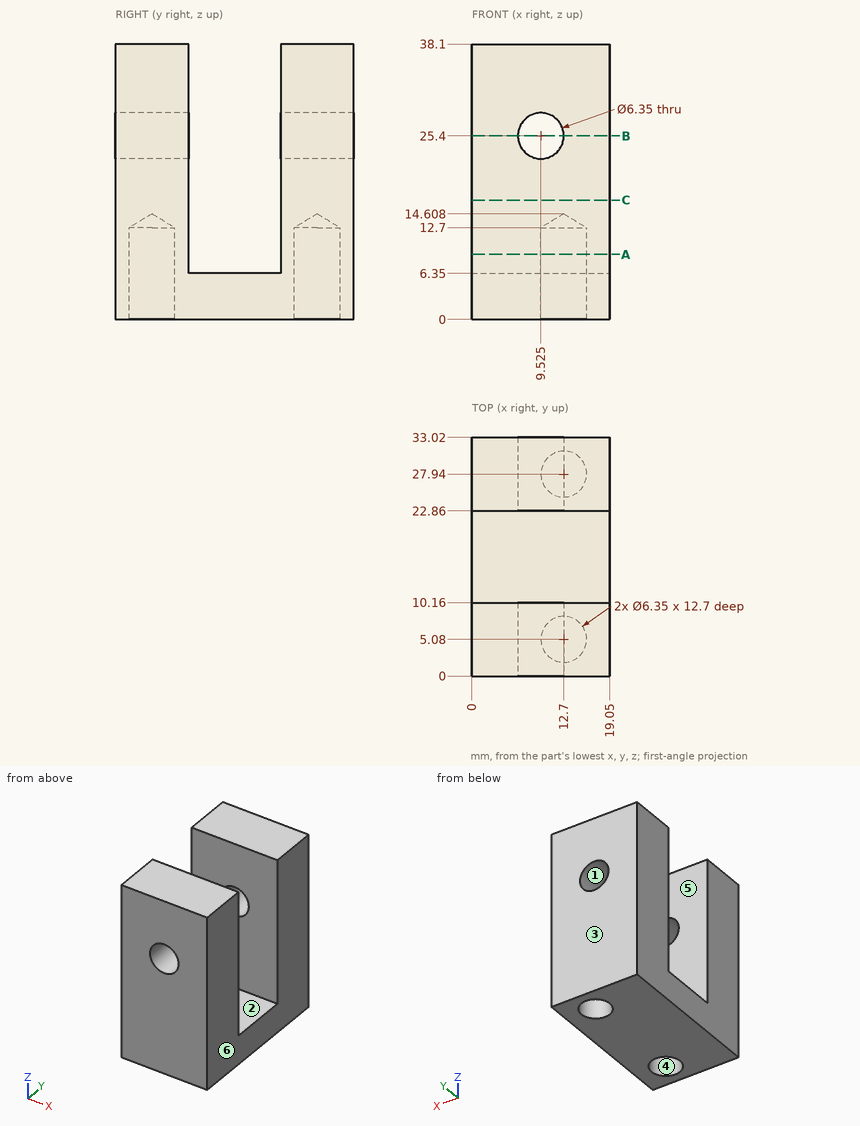
The figure shows three views and two pictorial views of one solid part (mm, origin at its lowest corner). Answer the questions. A direction names the side the tool comes from. Round coordinates to 2 decimals unless told otherwise and drop trailing zeros. Loops run counter-clockwise (first coordinate to the right, second up) from the corner with the lowest first, then second, coordinate; pieces in that order, holes last. Notation, with made-up numbers: (83.25, 63.5) - (136.25, 63.5) arc R19 ccw to (136.25, 71.5) - close; hole circle Ø1 at (42, 33). An arc over 180 degrees is marked (long way). Use one line per item in the form item = value. Start each with the question number.
(1) Find section A-A on z = 9. Give the number of separate pieces and of enclosed holes in the cut face, and give its area (3 significant figures).
(2) Find section C-C on z = 16.5. Determine the outline of the cut face in (x, y), and give its area (3 significant figures).
(3) Find section B-B on z = 25.4. Determine the outline of the cut face in (x, y), and give its area (3 significant figures).
(4) Determine the mould class of the marked faces 1, 2 and 3 for opening direction Y: +Y half, -Y half, draft (parallel to the pull), parting line (faces both ways), or undercut.
(5) A flat-ended cylindrical pin translates along its axis: P1, Ø5, axis at x = 12.7, y = 27.94, coming from the -Z side (1 decimal). Find the tip coordinate at first contact, or state that the pin passes through.
(6) Consider line 1 (Y direction, x = 12.7, z = 8) (1 decimal); line 2 (Y direction, x = 12.7, z = 5.5) (1 decimal); line 3 (Y direction, x = 4.5, z = 21). Determine where each line is inside the solid, lowest interval first.
(7) Which of the six approach directions +Z, -Z, +X, -X, +Y, -Y give full straight-line access (tool end or side, diameter ignored) to the marked faces 4, 5 and 6?
Answer list:
q1.separate_pieces = 2
q1.enclosed_holes = 2
q1.area = 324 mm^2
q2.outline = (0, 0) - (19.05, 0) - (19.05, 10.16) - (0, 10.16) - close; (0, 22.86) - (19.05, 22.86) - (19.05, 33.02) - (0, 33.02) - close
q2.area = 387 mm^2
q3.outline = (0, 0) - (6.35, 0) - (6.35, 10.16) - (0, 10.16) - close; (0, 22.86) - (6.35, 22.86) - (6.35, 33.02) - (0, 33.02) - close; (12.7, 0) - (19.05, 0) - (19.05, 10.16) - (12.7, 10.16) - close; (12.7, 22.86) - (19.05, 22.86) - (19.05, 33.02) - (12.7, 33.02) - close
q3.area = 258 mm^2
q4.face_1 = draft
q4.face_2 = undercut
q4.face_3 = +Y half
q5.P1 = 13.1
q6.line_1 = 0 to 1.9, 8.3 to 10.2, 22.9 to 24.8, 31.1 to 33
q6.line_2 = 0 to 1.9, 8.3 to 24.8, 31.1 to 33
q6.line_3 = 0 to 10.16, 22.86 to 33.02
q7.face_4 = -Z
q7.face_5 = +Z, +X, -X
q7.face_6 = +Z, -Z, +X, +Y, -Y
